Verification items for the finished model (mm, model axes). A direction names the side the tool comes from. Coordinates: 2 decimals unless noted, no trailing zeros. Write each loop counter-clockwise with the first axis right and the second up, starting at its lowest first coordinate (ties: lowest second). Pieces come first, ordered by that corner, then holes. Notation, with made-up numbers: M -16,68.5 L -4,68.5 A16 cw -4,99.5 Z; hole C 39,30 d11. An arc over 180 degrees is marked long. One line per item, written item: value.
Autodesk Inventor part; units mm, degrees
ref_plane "YZ Plane" through (0, 0, 0) normal (1, 0, 0) x (0, 1, 0)
ref_plane "XZ Plane" through (0, 0, 0) normal (0, 1, 0) x (-1, 0, 0)
ref_plane "XY Plane" through (0, 0, 0) normal (0, 0, 1) x (1, 0, 0)
sketch "Sketch1" plane through (0, 0, 0) normal (0, 0, 1) x (1, 0, 0)
  line L0 (0, -1.3086) -> (-76.2, -1.3086)
  line L1 (-76.2, -1.3086) -> (-76.2, 125.6914)
  line L2 (-76.2, 125.6914) -> (0, 125.6914)
  line L3 (0, 125.6914) -> (0, -1.3086)
  point P0 (0, 0)
  dimension "d0" = 76.2
  dimension "d1" = 127
extrude "Extrusion1" add sketch "Sketch1" along normal blind 175
sketch "Sketch2" plane through (0, 0, 175) normal (0, 0, 1) x (1, 0, 0)
  line L0 (-77.1669, 127.1854) -> (1.3323, 127.1854)
  line L1 (1.3323, 127.1854) -> (1.3323, -2.5417)
  line L2 (1.3323, -2.5417) -> (-77.1669, -2.5417)
  line L3 (-77.1669, -2.5417) -> (-77.1669, 127.1854)
  point P0 (0, 0)
extrude "Extrusion2" add sketch "Sketch2" along normal blind 7
fillet "Fillet1" radius 2 4 edges at (-76.2, -1.3086, 87.5) (0, -1.3086, 87.5) (-76.2, 125.6914, 87.5) (0, 125.6914, 87.5)
properties part number "jar" material "PMMA Plastic"
Item 1: Go/stop test with flat-tipped pins: P1, Ø3, axis at y = 113, z = 75.5, coming from the -X side; P2, Ø1.5, axis at x = -22.5, z = 130, coming from the +Y side; P3, Ø1.5, axis at y = 32.5, z = 19.5, coming from the +X side. Record where each tip stops, or that it passes through.
The answers:
P1: stops at x = -76.2
P2: stops at y = 125.69
P3: stops at x = 0
Item 2: Scan lines: line 1 (X direction, y = 82.5, z = 170); line 2 (Y direction, x = -22, z = 139). Record each from-to range of solid material in increasing order.
The answers:
line 1: x = -76.2 to 0
line 2: y = -1.31 to 125.69
Item 3: Access from +Z, -Z, +X, -X, +Y, -Y to the whole of each face (thin tool, end or side, straight path). Record for faces 1 (the face through (-38, -1.309, 86)), 2 (the face through (-76.2, 61, 86)), 3 (the face through (-39, 125.691, 86)), 4 (the face through (0, 63, 86)).
The answers:
face 1: -Z, +X, -X, -Y
face 2: -Z, -X, +Y, -Y
face 3: -Z, +X, -X, +Y
face 4: -Z, +X, +Y, -Y
Item 4: Cross-section at A-A, the plane x = -6. Enter the section's corners in (y, z), and give its area (3 significant figures).
The answers:
outline: M -2.54,175 L -1.31,175 L -1.31,0 L 125.69,0 L 125.69,175 L 127.19,175 L 127.19,182 L -2.54,182 Z
area: 23,100 mm²
Item 5: Cross-section at B-B, the plane y = 62. Enter the section's corners in (x, z).
The answers:
outline: M -77.17,175 L -76.2,175 L -76.2,0 L 0,0 L 0,175 L 1.33,175 L 1.33,182 L -77.17,182 Z
